The listing builds one solid part. Answer for the finished solid, in the listing's coordinates (mm). Give positions to 0.01 mm unless a question says otherwise; leave off trailing zeros.
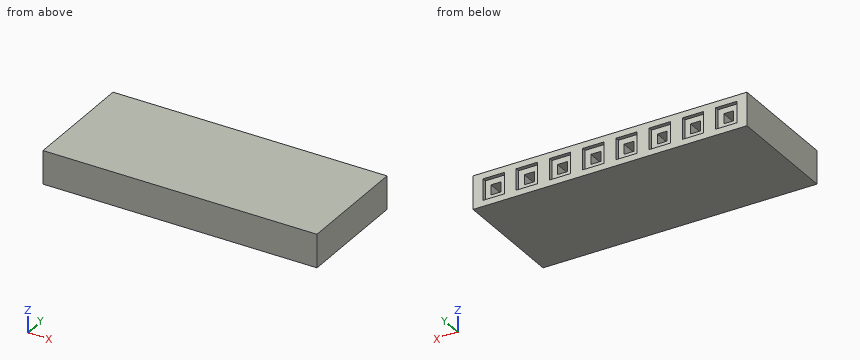
```python
from build123d import *

# Parameters (mm, degrees)
CROQUIS1_W              = 20.6
CROQUIS1_H              = 2.5
SALIENTE_EXTRUIR1_DEPTH = 8.7
CROQUIS3_W              = 1.6
CROQUIS3_H              = 1.6
CORTAR_EXTRUIR1_DEPTH   = 8.5
CROQUIS5_W              = 1.6
CROQUIS5_H              = 1.6
CROQUIS5_W_2            = 0.75
CROQUIS5_H_2            = 0.75
SALIENTE_EXTRUIR2_DEPTH = 8.2


with BuildPart() as part:
    # Croquis1 → Saliente-Extruir1 (new body)
    with BuildSketch(Plane(origin=(0, 0, 0), x_dir=(1, 0, 0), z_dir=(0, 1, 0))):
        Rectangle(CROQUIS1_W, CROQUIS1_H)
    extrude(amount=SALIENTE_EXTRUIR1_DEPTH)

    # Croquis3 → Cortar-Extruir1 (cut)
    with BuildSketch(Plane(origin=(0, 8.7, 0), x_dir=(1, 0, 0), z_dir=(0, 1, 0))):
        with Locations((-8.75, 0)):
            Rectangle(CROQUIS3_W, CROQUIS3_H)
        with Locations((-6.25, 0)):
            Rectangle(CROQUIS3_W, CROQUIS3_H)
        with Locations((-3.75, 0)):
            Rectangle(CROQUIS3_W, CROQUIS3_H)
        with Locations((-1.25, 0)):
            Rectangle(CROQUIS3_W, CROQUIS3_H)
        with Locations((1.25, 0)):
            Rectangle(CROQUIS3_W, CROQUIS3_H)
        with Locations((3.75, 0)):
            Rectangle(CROQUIS3_W, CROQUIS3_H)
        with Locations((6.25, 0)):
            Rectangle(CROQUIS3_W, CROQUIS3_H)
        with Locations((8.75, 0)):
            Rectangle(CROQUIS3_W, CROQUIS3_H)
    extrude(amount=-CORTAR_EXTRUIR1_DEPTH, mode=Mode.SUBTRACT)

    # Croquis5 → Saliente-Extruir2 (add)
    # profile 1 of 8: a face of its own
    with BuildSketch(Plane(origin=(0, 0.2, 0), x_dir=(1, 0, 0), z_dir=(0, 1, 0))):
        with Locations((-8.75, 0)):
            Rectangle(CROQUIS5_W, CROQUIS5_H)
        with Locations((-8.75, 0)):
            Rectangle(CROQUIS5_W_2, CROQUIS5_H_2, mode=Mode.SUBTRACT)
    # profile 2 of 8: a face of its own
    with BuildSketch(Plane(origin=(0, 0.2, 0), x_dir=(1, 0, 0), z_dir=(0, 1, 0))):
        with Locations((-6.25, 0)):
            Rectangle(CROQUIS5_W, CROQUIS5_H)
        with Locations((-6.25, 0)):
            Rectangle(CROQUIS5_W_2, CROQUIS5_H_2, mode=Mode.SUBTRACT)
    # profile 3 of 8: a face of its own
    with BuildSketch(Plane(origin=(0, 0.2, 0), x_dir=(1, 0, 0), z_dir=(0, 1, 0))):
        with Locations((-3.75, 0)):
            Rectangle(CROQUIS5_W, CROQUIS5_H)
        with Locations((-3.75, 0)):
            Rectangle(CROQUIS5_W_2, CROQUIS5_H_2, mode=Mode.SUBTRACT)
    # profile 4 of 8: a face of its own
    with BuildSketch(Plane(origin=(0, 0.2, 0), x_dir=(1, 0, 0), z_dir=(0, 1, 0))):
        with Locations((-1.25, 0)):
            Rectangle(CROQUIS5_W, CROQUIS5_H)
        with Locations((-1.25, 0)):
            Rectangle(CROQUIS5_W_2, CROQUIS5_H_2, mode=Mode.SUBTRACT)
    # profile 5 of 8: a face of its own
    with BuildSketch(Plane(origin=(0, 0.2, 0), x_dir=(1, 0, 0), z_dir=(0, 1, 0))):
        with Locations((1.25, 0)):
            Rectangle(CROQUIS5_W, CROQUIS5_H)
        with Locations((1.25, 0)):
            Rectangle(CROQUIS5_W_2, CROQUIS5_H_2, mode=Mode.SUBTRACT)
    # profile 6 of 8: a face of its own
    with BuildSketch(Plane(origin=(0, 0.2, 0), x_dir=(1, 0, 0), z_dir=(0, 1, 0))):
        with Locations((3.75, 0)):
            Rectangle(CROQUIS5_W, CROQUIS5_H)
        with Locations((3.75, 0)):
            Rectangle(CROQUIS5_W_2, CROQUIS5_H_2, mode=Mode.SUBTRACT)
    # profile 7 of 8: a face of its own
    with BuildSketch(Plane(origin=(0, 0.2, 0), x_dir=(1, 0, 0), z_dir=(0, 1, 0))):
        with Locations((6.25, 0)):
            Rectangle(CROQUIS5_W, CROQUIS5_H)
        with Locations((6.25, 0)):
            Rectangle(CROQUIS5_W_2, CROQUIS5_H_2, mode=Mode.SUBTRACT)
    # profile 8 of 8: a face of its own
    with BuildSketch(Plane(origin=(0, 0.2, 0), x_dir=(1, 0, 0), z_dir=(0, 1, 0))):
        with Locations((8.75, 0)):
            Rectangle(CROQUIS5_W, CROQUIS5_H)
        with Locations((8.75, 0)):
            Rectangle(CROQUIS5_W_2, CROQUIS5_H_2, mode=Mode.SUBTRACT)
    extrude(amount=SALIENTE_EXTRUIR2_DEPTH)


solid = part.part
```
1) Given P1, Ø1.5, axis at x = -7, z = 0, coming from the +Y side, flat-ended and moving along its own axis, determine where the tip first touches the part or whether it passes through.
Geometry says:
P1: stops at y = 8.7
2) Straight lines are drawn through the part: probe 1 along Z at (x, y) = (8.5, 8) (3 decimals); probe 2 along Y at (x, z) = (4.5, -0.5); probe 3 along Y at (x, z) = (-6.5, 0.2). For each, find the intervals that lie inside material, in ascending order.
Geometry says:
probe 1: z = -1.25 to -0.375, 0.375 to 1.25
probe 2: y = 0 to 8.4
probe 3: y = 0 to 0.2
3) Find section A-A (y = 4.25). Count the separate pieces of the cut face and the enclosed holes in it, then the cut area to 3 significant figures.
Geometry says:
separate pieces: 1
enclosed holes: 8
area: 47.0 mm2
